Design review of the part shown in the three views and the two pictorial views. Dimensions are in mm from the part's minimum x, y and z. A direction names the side the tool comes from. Give positions to 0.01 mm unless a question says otherwise; leave off trailing zeros. Order: outer loops, then holes, each group sorted by start corner. A loop starts at its lowest first (then second) coordinate and runs counter-clockwise, first axis right, second up. Notation, with made-up numbers: (74, -10) - (89, -10) arc R10 ccw to (89, -3) - close; hole circle Ø5 at (10.25, 40.5). An arc over 180 degrees is marked (long way). Put each result on its own line as item: value.
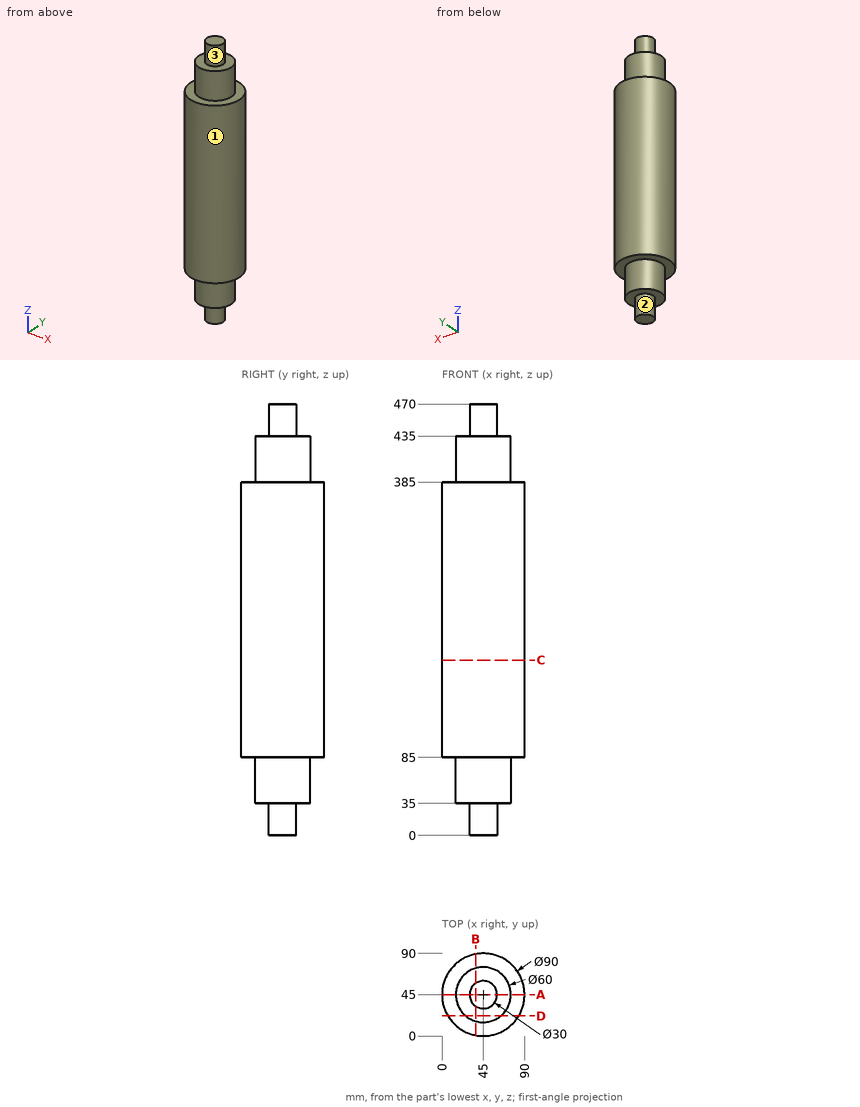
(1) Clearance check with flat-ended pins moving along their axes: pin 1 Ø10 at (y, z) = (38.5, 362.5) entering from +X (3 decimals); pin 2 Ø2 at (x, y) = (44.5, 21) entering from -Z; pin 3 Ø6 at (x, y) = (47, 52.5) entering from -Z; pin 4 Ø1 at (x, z) = (61.5, 264.5) entering from -Y. State where each tip first meets the part, or that it passes through.
The answers:
pin 1: x = 89.975
pin 2: z = 35
pin 3: z = 0
pin 4: y = 2.94
(2) Take a section at A-A, the plane y = 45. Write out the cut boundary in (x, z), then the cut area to 3 significant figures.
The answers:
outline: (0, 85) - (15, 85) - (15, 35) - (30, 35) - (30, 0) - (60, 0) - (60, 35) - (75, 35) - (75, 85) - (90, 85) - (90, 385) - (75, 385) - (75, 435) - (60, 435) - (60, 470) - (30, 470) - (30, 435) - (15, 435) - (15, 385) - (0, 385) - close
area: 35,100 mm^2
(3) Wall thickness on L1, parallel to Z at x = 72, y = 33; L2, parallel to Z at x = 9, y = 58; L3, parallel to Y at x = 47, z = 277.5: over which ranges is each line inside the solid? List them lowest first.
The answers:
L1: 35 to 435
L2: 85 to 385
L3: 0.04 to 89.96
(4) For the marked faces 1, 2 and 3, list the 3-axis set-ups (+Z, -Z, +X, -X, +Y, -Y) from which the entire face can be reached by the end or side of a thin tool; tool diameter is ignored.
The answers:
face 1: +Z, -Z
face 2: -Z
face 3: +Z
(5) Take a section at D-D, the plane y = 22. Write out the cut boundary in (x, z).
The answers:
outline: (6.32, 85) - (25.74, 85) - (25.74, 35) - (64.26, 35) - (64.26, 85) - (83.68, 85) - (83.68, 385) - (64.26, 385) - (64.26, 435) - (25.74, 435) - (25.74, 385) - (6.32, 385) - close
(6) Take a section at C-C, the plane z = 191. Write out the cut boundary in (x, y), then the cut area to 3 significant figures.
The answers:
outline: circle Ø90 at (45, 45)
area: 6,360 mm^2
(7) Take a section at B-B, the plane x = 36.5. Write out the cut boundary in (y, z), then the cut area to 3 significant figures.
The answers:
outline: (0.81, 85) - (16.23, 85) - (16.23, 35) - (32.64, 35) - (32.64, 0) - (57.36, 0) - (57.36, 35) - (73.77, 35) - (73.77, 85) - (89.19, 85) - (89.19, 385) - (73.77, 385) - (73.77, 435) - (57.36, 435) - (57.36, 470) - (32.64, 470) - (32.64, 435) - (16.23, 435) - (16.23, 385) - (0.81, 385) - close
area: 34,000 mm^2
